Part model, mm, in its own coordinate system. Face numbers are marked on the shaded views. A direction names the side the tool comes from. Give positions to 0.01 mm unless a question says otherwise; leave off trailing zeros. Order: outer loops, then holes, each group sorted by start corner. A loop starts at its lowest first (then second) coordinate and runs counter-clockwise, first axis right, second up. Notation, with made-up numbers: M -31,-15 L 5,-15 A14 cw 5,-7 Z; hole C 75.5,38 d7. An arc over 180 degrees is marked long. One line per question, with ' | ' between items.
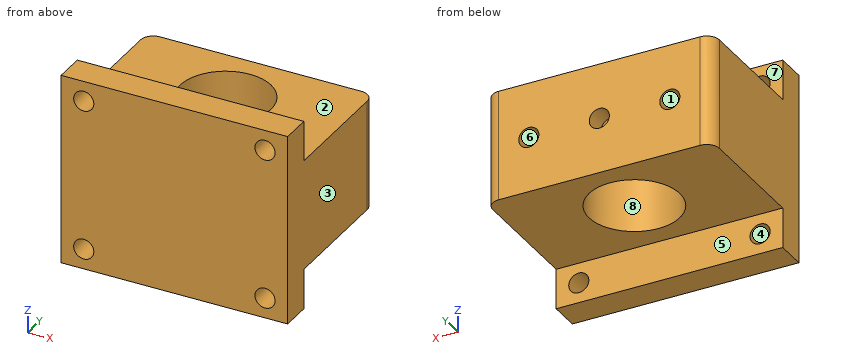
```python
from build123d import *

# Parameters (mm, degrees)
SKETCH1_R               = 9
BOSS_EXTRUDE1_DEPTH     = 11
SKETCH1_3_W             = 45
SKETCH1_3_H             = 6
BOSS_EXTRUDE2_DEPTH     = 19
SKETCH2_R               = 2
CUT_EXTRUDE1_DEPTH      = 40.284220751
CUT_EXTRUDE2_REACH      = 45.489
CUT_EXTRUDE2_END_RADIUS = 9
SKETCH3_R               = 2
SKETCH3_3_R             = 2
CUT_EXTRUDE3_DEPTH      = 20


with BuildPart() as part:
    # Sketch1 → Boss-Extrude1 (new, symmetric)
    with BuildSketch(Plane.XY):
        with BuildLine():
            Line((-20, 13), (20, 13))
            ThreePointArc((20, 13), (21.767766953, 12.267766953), (22.5, 10.5))
            Line((22.5, 10.5), (22.5, -13))
            Line((22.5, -13), (-22.5, -13))
            Line((-22.5, -13), (-22.5, 10.5))
            ThreePointArc((-22.5, 10.5), (-21.767766953, 12.267766953), (-20, 13))
        make_face()
        Circle(SKETCH1_R, mode=Mode.SUBTRACT)
    extrude(amount=BOSS_EXTRUDE1_DEPTH, both=True)

    # Sketch1<3> → Boss-Extrude2 (add, symmetric)
    with BuildSketch(Plane.XY):
        with Locations((0, -16)):
            Rectangle(SKETCH1_3_W, SKETCH1_3_H)
    extrude(amount=BOSS_EXTRUDE2_DEPTH, both=True)

    # Sketch2 → Cut-Extrude1 (cut, through all)
    with BuildSketch(Plane(origin=(0, -13, 0), x_dir=(1, 0, 0), z_dir=(0, 1, 0))):
        with Locations(Location((-18, -15, 0), (0, 0, 270))):
            Circle(SKETCH2_R)
        with Locations(Location((18, -15, 0), (0, 0, 90))):
            Circle(SKETCH2_R)
        with Locations(Location((18, 15, 0), (0, 0, 270))):
            Circle(SKETCH2_R)
        with Locations(Location((-18, 15, 0), (0, 0, 90))):
            Circle(SKETCH2_R)
    extrude(amount=-CUT_EXTRUDE1_DEPTH, mode=Mode.SUBTRACT)

    # Cut-Extrude2: up to this cylinder (the profile starts outside it)
    cut_extrude2_end = Plane(origin=(0, 0, 0), z_dir=(0, 0, -1)) * Cylinder(CUT_EXTRUDE2_END_RADIUS, 109.978, mode=Mode.PRIVATE)
    # Sketch3 → Cut-Extrude2 (cut, up to the surface)
    with BuildSketch(Plane(origin=(0, 13, 0), x_dir=(1, 0, 0), z_dir=(0, 1, 0)), mode=Mode.PRIVATE) as cut_extrude2_sk1:
        with Locations(Location((0, 0, 0), (0, 0, 270))):
            Circle(SKETCH3_R)
    cut_extrude2_tool1 = extrude(cut_extrude2_sk1.sketch, amount=-CUT_EXTRUDE2_REACH, mode=Mode.PRIVATE) - cut_extrude2_end
    add(cut_extrude2_tool1.solids().sort_by_distance((0, 13, 0))[0], mode=Mode.SUBTRACT)

    # Sketch3<3> → Cut-Extrude3 (cut)
    with BuildSketch(Plane(origin=(0, 13, 0), x_dir=(1, 0, 0), z_dir=(0, 1, 0))):
        with Locations(Location((-14, 0, 0), (0, 0, 270))):
            Circle(SKETCH3_3_R)
    cut_extrude3 = extrude(amount=-CUT_EXTRUDE3_DEPTH, mode=Mode.SUBTRACT)

    # Mirror1: Cut-Extrude3 across plane
    add(cut_extrude3.mirror(Plane(origin=(0, 0, 0), x_dir=(0, 0, 1), z_dir=(1, 0, 0))), mode=Mode.SUBTRACT)


solid = part.part
```
1. Slice it at B-B on x = 0. Give the cut face in (y, z).
Worked out:
outline: M -19,-19 L -13,-19 L -13,-11 L -9,-11 L -9,11 L -13,11 L -13,19 L -19,19 Z; M 9,-11 L 13,-11 L 13,-2 L 9,-2 Z; M 9,2 L 13,2 L 13,11 L 9,11 Z
2. Slice it at A-A on y = 0. Give the cut face in (x, z).
Worked out:
outline: M -22.5,-11 L -9,-11 L -9,11 L -22.5,11 Z; M 9,-11 L 22.5,-11 L 22.5,11 L 9,11 Z; hole C -14,0 d4; hole C 14,0 d4
3. Probe L1, parallel to X at y = -15.2, z = 15; L2, parallel to X at y = 7.5, z = 0; L3, parallel to X at y = -18, z = 13.5. List the from-to ranges inside material, lowest first. Write a range as from..to.
Worked out:
L1: x = -22.5..-20, -16..16, 20..22.5 | L2: x = -22.5..-16, -12..-4.97, 4.97..12, 16..22.5 | L3: x = -22.5..-19.32, -16.68..16.68, 19.32..22.5
4. Slice it at C-C on z = -15. Give the cut face in (x, y).
Worked out:
outline: M -22.5,-19 L -20,-19 L -20,-13 L -22.5,-13 Z; M -16,-19 L 16,-19 L 16,-13 L -16,-13 Z; M 20,-19 L 22.5,-19 L 22.5,-13 L 20,-13 Z
5. Drop flat-ended pins along their axis: pin 1 (4 mm diameter, centred on x = -2, z = -13.5, fed in from +Y); pin 2 (1.2 mm diameter, centred on x = 13.5, z = 1, fed in from +Y); pin 3 (4 mm diameter, centred on x = 5, y = -10, fed in from -Z). Give the stop position or say it passes through.
Worked out:
pin 1: stops at y = -13 | pin 2: stops at y = -7 | pin 3: stops at z = -11
6. Tool access for the marked faces 5, 6, 7 and 8: list every direction of +Z, -Z, +X, -X, +Y, -Y with a clear straight run to the whole face (end or side of a thin tool).
Worked out:
face 5: -Z, +X, -X, +Y | face 6: +Y | face 7: +Z, +X, -X, +Y | face 8: +Z, -Z
7. Slice it at D-D on x = -7.5. Give the cut face in (y, z), then the cut area to 3 significant figures.
Worked out:
outline: M -19,-19 L -13,-19 L -13,-11 L -4.97,-11 L -4.97,11 L -13,11 L -13,19 L -19,19 Z; M 4.97,-11 L 13,-11 L 13,11 L 4.97,11 Z | area: 581 mm2
8. Mould opens along X. For the marked faces 1, 2, 3 and 4 say: released by +X, released by -X, zero draft, split by the parting line, or undercut.
Worked out:
face 1: undercut | face 2: zero draft | face 3: released by +X | face 4: undercut
